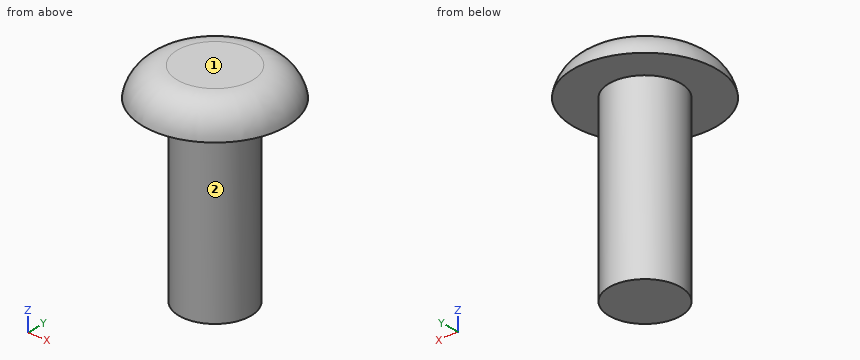
```python
from build123d import *

# Parameters (mm, degrees)
F0_R     = 6.35
F1_DEPTH = 2.54
F3_R     = 3.175
F4_DEPTH = 15.875


# Not quite as in the source:
# - a fillet or chamfer that OpenCascade refuses, or shapes differently, is made with other operations: its cross-section is extruded or revolved along the edge and cut away or added


with BuildPart() as f1:
    # F0 (on Top) → F1 (new body)
    with BuildSketch(Plane.XY):
        Circle(F0_R)
    extrude(amount=F1_DEPTH)

    # F2: fillet of radius 3.0660512242 on 1 edges, made by hand

    # F2_s1 → F2_t2 (revolve, cut)
    with BuildSketch(Plane.XZ):
        with BuildLine():
            ThreePointArc((6.35, 0), (5.3027068749, 1.8206027884), (3.3294139279, 2.54))
            Line((3.3294139279, 2.54), (6.35, 2.54))
            Line((6.35, 2.54), (6.35, 0))
        make_face()
    revolve(axis=Axis((0, 0, 2.54), (0, 0, 1)), mode=Mode.SUBTRACT)

    # F3 (on face) → F4 (join)
    with BuildSketch(Plane(origin=(0, 0, 0), x_dir=(1, 0, 0), z_dir=(0, 0, -1))):
        Circle(F3_R)
    extrude(amount=F4_DEPTH)


solid = f1.part
```
The model under review builds one solid part; all positions refer to its coordinate system, in mm. Face numbers are marked on the shaded views. A direction names the side the tool comes from. Give positions to 0.01 mm unless a question says otherwise; leave off trailing zeros. Write each loop counter-clockwise with the first axis right and the second up, starting at its lowest first coordinate (ties: lowest second). Pieces come first, ordered by that corner, then holes. Notation, with made-up numbers: M 79,46 L 110,46 A26 cw 110,75 Z; hole C -18,75 d10. An arc over 180 degrees is marked long. Answer in a Markdown table with one row per item.
Item 1: Add section C-C on z = -14. Give the boundary of the cut face in (x, y) (3 decimals), plus the area to 3 significant figures.
Check sheet entries:
| item | result |
|---|---|
| outline | C 0,0 d6.35 |
| area | 31.7 mm2 |
Item 2: Tool access review of the marked faces 1 and 2: name each direction out of +Z, -Z, +X, -X, +Y, -Y from which nothing blocks a thin tool from reaching the whole face with its end or side.
Check sheet entries:
| item | result |
|---|---|
| face 1 | +Z, +X, -X, +Y, -Y |
| face 2 | -Z |
Item 3: Add section A-A on y = 0. Give the boundary of the cut face in (x, z) (3 decimals), plus the area to 3 significant figures.
Check sheet entries:
| item | result |
|---|---|
| outline | M -6.35,0 L -3.175,0 L -3.175,-15.875 L 3.175,-15.875 L 3.175,0 L 6.35,0 A3.066 ccw 3.329,2.54 L -3.329,2.54 A3.066 ccw Z |
| area | 129 mm2 |
Item 4: For line 1 along X through (y, z) = (-1.5, -13); line 2 along X through (y, z) = (-0.25, -12); line 3 along Z through (x, y) = (2.25, 3), list the stretches that pass through material, from the lowest coordinate up.
Check sheet entries:
| item | result |
|---|---|
| line 1 | -2.8 to 2.8 |
| line 2 | -3.17 to 3.17 |
| line 3 | 0 to 2.51 |
Item 5: Add section D-D on z = 1. Give the boundary of the cut face in (x, y).
Check sheet entries:
| item | result |
|---|---|
| outline | C 0,0 d11.98 |
Item 6: For P1, Ø1, axis at y = 2.5, z = -9, coming from the +X side; P2, Ø4, axis at y = 3, z = -1, coming from the +X side; P3, Ø6, axis at x = 0, z = -6, coming from the +Y side (3 decimals), all flat-tipped, find the tip position at first contact; note any pin that passes through.
Check sheet entries:
| item | result |
|---|---|
| P1 | x = 2.47 |
| P2 | x = 6.22 |
| P3 | y = 3.175 |
